from build123d import *

# Parameters (mm, degrees)
F3_D            = 3
F3_CBORE_D      = 5
F3_CBORE_DEPTH  = 4
F4_D            = 2.5
F4_CBORE_D      = 4
F4_CBORE_DEPTH  = 5
F4_COPIES_COUNT = 4
F5_W            = 2
F5_H            = 35
F5_H_2          = 11.5
F6_DEPTH        = 5


# Not quite as in the source:
# - a pattern or mirror of a feature is missing from the dataset's text; its kind, count and spacing are read off the source's solid


with BuildPart() as f1:
    # F0 (on Front) → F1 (revolve)
    with BuildSketch(Plane.XZ):
        Polygon((0, 8), (0, 0), (8, 0), (8, -1), (9, -1), (9, 0), (16, 0), (16, 5.44932126), (4, 8), align=None)
    revolve(axis=Axis((0, 0, 4), (0, 0, 1)))

    # F3 (through all)
    with Locations(Plane.XY.offset(8)):
        with Locations((0, 0)):
            CounterBoreHole(F3_D / 2, F3_CBORE_D / 2, F3_CBORE_DEPTH)

    # F4 (through all)
    with Locations(Plane.XY.offset(8)):
        with Locations((-8.1317279836, 8.1317279836)):
            f4 = CounterBoreHole(F4_D / 2, F4_CBORE_D / 2, F4_CBORE_DEPTH)

    # F4_copies: F4 ×4 about axis
    f4_copies_axis = Axis((0, 0, 0), (0, 0, 1))
    for i in range(1, F4_COPIES_COUNT):
        add(f4.rotate(f4_copies_axis, i * 360 / F4_COPIES_COUNT), mode=Mode.SUBTRACT)

    # F5 (on face) → F6 (cut)
    with BuildSketch(Plane.XY.offset(8)):
        with Locations((-4, 0)):
            Rectangle(F5_W, F5_H)
        with Locations((-8.4, 0)):
            Rectangle(F5_W, F5_H)
        with Locations((-12.8, 0)):
            Rectangle(F5_W, F5_H)
        with Locations((4, 0)):
            Rectangle(F5_W, F5_H)
        with Locations((8.4, 0)):
            Rectangle(F5_W, F5_H)
        with Locations((12.8, 0)):
            Rectangle(F5_W, F5_H)
        with Locations((0, 11.75)):
            Rectangle(F5_W, F5_H_2)
        with Locations((0, -11.75)):
            Rectangle(F5_W, F5_H_2)
    extrude(amount=-F6_DEPTH, mode=Mode.SUBTRACT)


solid = f1.part
Verification items for the finished model (mm, model axes). A direction names the side the tool comes from. Coordinates: 2 decimals unless noted, no trailing zeros. Order: outer loops, then holes, each group sorted by start corner. A loop starts at its lowest first (then second) coordinate and runs counter-clockwise, first axis right, second up. Notation, with made-up numbers: M 3.25,33.5 L 60.25,33.5 A23 ccw 60.25,48.5 Z; hole C 88.25,79 d8. An arc over 180 degrees is marked long. Return JSON: item names as keys, results as strings.
1) Gauge pin test, flat ends, axial feed: pin 1 (6 mm diameter, centred on x = -6.5, y = 1.5, fed in from +Z); pin 2 (1 mm diameter, centred on y = 2.5, z = 2.5, fed in from +X); pin 3 (2 mm diameter, centred on x = 8.13, y = 8.13, fed in from -Z); pin 4 (1.5 mm diameter, centred on y = 1, z = 4.5, fed in from -X). Record the tip position at first contact, or that the pin passes through.
Answer list:
{"pin 1": "z = 7.79", "pin 2": "x = 15.87", "pin 3": "through", "pin 4": "x = -16"}
2) Cross-section at A-A, the plane x = 0. Record the boundary of the cut face in (y, z).
Answer list:
{"outline": "M -16,0 L -9,0 L -9,-1 L -8,-1 L -8,0 L -1.5,0 L -1.5,4 L -2.5,4 L -2.5,8 L -4,8 L -6,7.57 L -6,3 L -16,3 Z; M 1.5,0 L 8,0 L 8,-1 L 9,-1 L 9,0 L 16,0 L 16,3 L 6,3 L 6,7.57 L 4,8 L 2.5,8 L 2.5,4 L 1.5,4 Z"}
3) Cross-section at B-B, the plane x = -4. Record the boundary of the cut face in (y, z), and give its area (3 significant figures).
Answer list:
{"outline": "M -15.49,0 L -8.06,0 L -8.06,-1 L -6.93,-1 L -6.93,0 L 6.93,0 L 6.93,-1 L 8.06,-1 L 8.06,0 L 15.49,0 L 15.49,3 L -15.49,3 Z", "area": "95.2 mm2"}
4) Release check for a two-part mould opening along Y. For faces 4 (the conical face through (-1.34, 7.181, 7.297)), 5 (the flat face through (0, 11, 3)), 6 (the cylindrical face through (-0.54, -2.44, 6.03)) record: +Y half, -Y half, draft (parallel to the pull), parting line (faces both ways), or undercut.
Answer list:
{"face 4": "+Y half", "face 5": "draft", "face 6": "undercut"}
5) Access from +Z, -Z, +X, -X, +Y, -Y to the whole of each face (thin tool, end or side, straight path). Record for faces 1 (the cylindrical face through (10.13, -8.16, 4.73)), 2 (the conical face through (10.45, -0.14, 6.63)), 3 (the flat face through (4, 0, 3)).
Answer list:
{"face 1": "+Z", "face 2": "+Z, +X", "face 3": "+Z, +Y, -Y"}
6) Thickness scan on L1, parallel to X at y = 14, z = 4.5; L2, parallel to X at y = 5, z = 6.75; L3, parallel to X at y = 2, z = 6. Record the ranges inside material, lowest first. Write a range as [from, to].
Answer list:
{"L1": "[-7.4, -5], [-3, -1], [1, 3], [5, 7.4]", "L2": "[-7.4, -5], [-3, 3], [5, 7.4]", "L3": "[-11.8, -9.4], [-7.4, -5], [-3, -1.5], [1.5, 3], [5, 7.4], [9.4, 11.8]"}
